Can you work these out from the model? Positions are in its coordinate system, mm. Face numbers are marked on the shaded views. A direction names the side the tool comes from. Round coordinates to 2 decimals unless told otherwise and drop trailing zeros. Order: outer loops, then holes, each group sorted by start corner. A loop starts at its lowest first (then second) coordinate and runs counter-clockwise, first axis right, second up. Notation, with made-up numbers: M -5,62 L 18,62 A4 cw 18,66 Z; hole C -30,12 d11. An arc over 180 degrees is marked long. One line per question, with ' | ' between items.
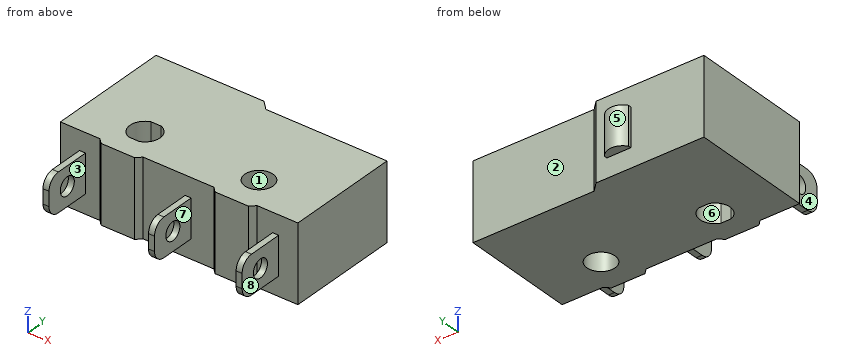
```python
from build123d import *

# Parameters (mm, degrees)
CUT_EXTRUDE1_START       = -3.2
CUT_EXTRUDE1_OUTLINE_R   = 1.175
CUT_EXTRUDE1_DEPTH       = 6.4
CUT_EXTRUDE1_START_2     = -1.6
CUT_EXTRUDE1_2_OUTLINE_W = 0.5
CUT_EXTRUDE1_2_OUTLINE_H = 3.9
CUT_EXTRUDE1_2_DEPTH     = 0.8499999
CUT_EXTRUDE1_START_3     = 0.7500001
CUT_EXTRUDE1_3_OUTLINE_W = 0.5
CUT_EXTRUDE1_3_OUTLINE_H = 3.9
CUT_EXTRUDE1_3_DEPTH     = 0.8499999
CUT_EXTRUDE1_4_DEPTH     = 3.2
CUT_EXTRUDE1_START_4     = -13
CUT_EXTRUDE1_5_DEPTH     = 0.5
CUT_EXTRUDE1_START_5     = -4.2
CUT_EXTRUDE1_6_DEPTH     = 0.5
CUT_EXTRUDE1_START_6     = 3.1
CUT_EXTRUDE1_7_DEPTH     = 0.5
FILLET1_R                = 1


with BuildPart() as part:
    # Cut-Extrude1: read off the stored shape, not the designer's step
    # Cut-Extrude1 outline → Cut-Extrude1 (new body)
    with BuildSketch(Plane.XY.offset(CUT_EXTRUDE1_START)):
        Polygon((-14.6, -2.5), (-11.3, -2.5), (-10.9, -2.9), (-8.1, -2.9), (-7.7, -2.5), (-1.8, -2.5), (-1.4, -2.9), (1.4, -2.9), (1.8, -2.5), (5.2, -2.5), (5.2, 7), (-4.9, 7), (-5.6, 7.7), (-14.6, 7.7), align=None)
        with BuildLine():
            ThreePointArc((-9.926468053, -1.175), (-10.75, 0), (-9.926468053, 1.175))
            Line((-9.926468053, 1.175), (-9.073531947, 1.175))
            ThreePointArc((-9.073531947, 1.175), (-8.25, 0), (-9.073531947, -1.175))
            Line((-9.073531947, -1.175), (-9.926468053, -1.175))
        make_face(mode=Mode.SUBTRACT)
        Circle(CUT_EXTRUDE1_OUTLINE_R, mode=Mode.SUBTRACT)
    extrude(amount=CUT_EXTRUDE1_DEPTH)

    # Cut-Extrude1 2 outline → Cut-Extrude1 2 (add)
    with BuildSketch(Plane.XY.offset(CUT_EXTRUDE1_START_2)):
        with Locations((-12.75, -4.45)):
            Rectangle(CUT_EXTRUDE1_2_OUTLINE_W, CUT_EXTRUDE1_2_OUTLINE_H)
        with Locations((-3.95, -4.45)):
            Rectangle(CUT_EXTRUDE1_2_OUTLINE_W, CUT_EXTRUDE1_2_OUTLINE_H)
        with BuildLine():
            Line((-8.5, 7.936178156), (-8.5, 7.7))
            Line((-8.5, 7.7), (-6.5, 7.7))
            Line((-6.5, 7.7), (-6.5, 7.936178156))
            ThreePointArc((-6.5, 7.936178156), (-7.5, 8.472853198), (-8.5, 7.936178156))
        make_face()
        with Locations((3.35, -4.45)):
            Rectangle(CUT_EXTRUDE1_2_OUTLINE_W, CUT_EXTRUDE1_2_OUTLINE_H)
    extrude(amount=CUT_EXTRUDE1_2_DEPTH)

    # Cut-Extrude1 3 outline → Cut-Extrude1 3 (add)
    with BuildSketch(Plane.XY.offset(CUT_EXTRUDE1_START_3)):
        with Locations((-12.75, -4.45)):
            Rectangle(CUT_EXTRUDE1_3_OUTLINE_W, CUT_EXTRUDE1_3_OUTLINE_H)
        with Locations((-3.95, -4.45)):
            Rectangle(CUT_EXTRUDE1_3_OUTLINE_W, CUT_EXTRUDE1_3_OUTLINE_H)
        with BuildLine():
            Line((-8.5, 7.936178156), (-8.5, 7.7))
            Line((-8.5, 7.7), (-6.5, 7.7))
            Line((-6.5, 7.7), (-6.5, 7.936178156))
            ThreePointArc((-6.5, 7.936178156), (-7.5, 8.472853198), (-8.5, 7.936178156))
        make_face()
        with Locations((3.35, -4.45)):
            Rectangle(CUT_EXTRUDE1_3_OUTLINE_W, CUT_EXTRUDE1_3_OUTLINE_H)
    extrude(amount=CUT_EXTRUDE1_3_DEPTH)

    # Cut-Extrude1 4 outline → Cut-Extrude1 4 (add)
    with BuildSketch(Plane.XY.offset(CUT_EXTRUDE1_START_2)):
        with BuildLine():
            Line((-8.5, 7.936178156), (-8.5, 7.7))
            Line((-8.5, 7.7), (-6.5, 7.7))
            Line((-6.5, 7.7), (-6.5, 7.936178156))
            ThreePointArc((-6.5, 7.936178156), (-7.5, 8.472853198), (-8.5, 7.936178156))
        make_face()
    extrude(amount=CUT_EXTRUDE1_4_DEPTH)

    # Cut-Extrude1 5 outline → Cut-Extrude1 5 (add)
    with BuildSketch(Plane.YZ.offset(CUT_EXTRUDE1_START_4)):
        with BuildLine():
            Line((-4.45, 0.75), (-6.4, 0.7500001))
            Line((-6.4, 0.7500001), (-6.4, -0.7500001))
            Line((-6.4, -0.7500001), (-4.45, -0.75))
            ThreePointArc((-4.45, -0.75), (-5.2, 0), (-4.45, 0.75))
        make_face()
        with BuildLine():
            Line((-2.5, 0.7500001), (-4.45, 0.75))
            ThreePointArc((-4.45, 0.75), (-3.7, 0), (-4.45, -0.75))
            Line((-4.45, -0.75), (-2.5, -0.7500001))
            Line((-2.5, -0.7500001), (-2.5, 0.7500001))
        make_face()
    extrude(amount=CUT_EXTRUDE1_5_DEPTH)

    # Cut-Extrude1 6 outline → Cut-Extrude1 6 (add)
    with BuildSketch(Plane.YZ.offset(CUT_EXTRUDE1_START_5)):
        with BuildLine():
            Line((-4.45, 0.75), (-6.4, 0.7500001))
            Line((-6.4, 0.7500001), (-6.4, -0.7500001))
            Line((-6.4, -0.7500001), (-4.45, -0.75))
            ThreePointArc((-4.45, -0.75), (-5.2, 0), (-4.45, 0.75))
        make_face()
        with BuildLine():
            Line((-2.5, 0.7500001), (-4.45, 0.75))
            ThreePointArc((-4.45, 0.75), (-3.7, 0), (-4.45, -0.75))
            Line((-4.45, -0.75), (-2.5, -0.7500001))
            Line((-2.5, -0.7500001), (-2.5, 0.7500001))
        make_face()
    extrude(amount=CUT_EXTRUDE1_6_DEPTH)

    # Cut-Extrude1 7 outline → Cut-Extrude1 7 (add)
    with BuildSketch(Plane.YZ.offset(CUT_EXTRUDE1_START_6)):
        with BuildLine():
            Line((-4.45, 0.75), (-6.4, 0.7500001))
            Line((-6.4, 0.7500001), (-6.4, -0.7500001))
            Line((-6.4, -0.7500001), (-4.45, -0.75))
            ThreePointArc((-4.45, -0.75), (-5.2, 0), (-4.45, 0.75))
        make_face()
        with BuildLine():
            Line((-2.5, 0.7500001), (-4.45, 0.75))
            ThreePointArc((-4.45, 0.75), (-3.7, 0), (-4.45, -0.75))
            Line((-4.45, -0.75), (-2.5, -0.7500001))
            Line((-2.5, -0.7500001), (-2.5, 0.7500001))
        make_face()
    extrude(amount=CUT_EXTRUDE1_7_DEPTH)

    # Fillet1
    fillet1_edges = [part.edges().sort_by_distance(p)[0] for p in [
        (-12.75, -6.4, 1.6),
        (-12.75, -6.4, -1.6),
        (-3.95, -6.4, -1.6),
        (-3.95, -6.4, 1.6),
        (3.35, -6.4, -1.6),
        (3.35, -6.4, 1.6),
    ]]
    fillet(fillet1_edges, radius=FILLET1_R)


solid = part.part
```
(1) On a 3-axis mill with a long thin cutter (end or side, diameter ignored), from which of +Z, -Z, +X, -X, +Y, -Y can I reach the whole of each face in a straight line? I mean the marked faces 4, 5, 6, 7 and 8. Say none if no direction works.
Final values:
face 4: +Z, -Z, -X, -Y | face 5: +Z, -Z, +Y | face 6: +Z, -Z | face 7: +Z, -Z, -Y | face 8: +Z, -Z, +X, -Y
(2) If we section it at A-A on y = -4.45: Please give me the cut outline in (x, z), plus the area to 3 significant figures.
Final values:
outline: M -13,-1.6 L -12.5,-1.6 L -12.5,-0.75 L -13,-0.75 Z; M -13,0.75 L -12.5,0.75 L -12.5,1.6 L -13,1.6 Z; M -4.2,-1.6 L -3.7,-1.6 L -3.7,-0.75 L -4.2,-0.75 Z; M -4.2,0.75 L -3.7,0.75 L -3.7,1.6 L -4.2,1.6 Z; M 3.1,-1.6 L 3.6,-1.6 L 3.6,-0.75 L 3.1,-0.75 Z; M 3.1,0.75 L 3.6,0.75 L 3.6,1.6 L 3.1,1.6 Z | area: 2.55 mm^2
(3) If we section it at C-C on z = 0: State how many separate pieces and enclosed holes the cut face has, plus the area to 3 significant figures.
Final values:
separate pieces: 4 | enclosed holes: 2 | area: 193 mm^2
(4) If we section it at B-B on x = 0: Please give me the cut outline in (y, z) (3 decimals), plus the area to 3 significant figures.
Final values:
outline: M -2.9,-3.2 L -1.175,-3.2 L -1.175,3.2 L -2.9,3.2 Z; M 1.175,-3.2 L 7,-3.2 L 7,3.2 L 1.175,3.2 Z | area: 48.3 mm^2
(5) Will these pins go through, and if not, where does the flat tip stop? pin 1 Ø2.5 at (y, z) = (-4, 0) entering from -X; pin 2 Ø1.9 at (x, y) = (0, 0) entering from -Z (3 decimals); pin 3 Ø1.9 at (x, z) = (-0.5, -1.5) entering from +Y; pin 4 Ø1.8 at (x, z) = (-5.5, -0.5) entering from -Y.
Final values:
pin 1: x = -13 | pin 2: through | pin 3: y = 7 | pin 4: y = -2.5
(6) Thinking about a two-plate mould opening in Y: for the marked faces 1, 2 and 3, which applies, released by +Y, released by -Y, zero draft, split by the parting line, or undercut?
Final values:
face 1: undercut | face 2: released by +Y | face 3: zero draft
(7) Please list where these lines run through material, in increasing order: probe 1 along Z at (x, y) = (3.5, -4.45); probe 2 along Y at (x, z) = (-8.5, -2.25); probe 3 along X at (y, z) = (1, 0.25). Write a range as [from, to].
Final values:
probe 1: [-1.6, -0.75], [0.75, 1.6] | probe 2: [-2.9, -0.75], [0.75, 7.7] | probe 3: [-14.6, -10.25], [-8.75, -0.62], [0.62, 5.2]
